Autodesk Inventor part; units mm, degrees
ref_plane "YZ Plane" through (0, 0, 0) normal (1, 0, 0) x (0, 1, 0)
ref_plane "XZ Plane" through (0, 0, 0) normal (0, 1, 0) x (-1, 0, 0)
ref_plane "XY Plane" through (0, 0, 0) normal (0, 0, 1) x (1, 0, 0)
sketch "Sketch1" plane through (0, 0, 0) normal (0, 1, 0) x (-1, 0, 0)
  line L0 (0, 0) -> (0, -100)
  line L1 (0, -100) -> (20, -100)
  line L2 (20, -100) -> (20, 0)
  line L3 (20, 0) -> (0, 0)
  point P0 (10, -5)
  point P1 (10, -95)
  dimension "d0" = 100
  dimension "d1" = 20
  dimension "d2" = 90
  dimension "d3" = 5
extrude "Extrusion1" add sketch "Sketch1" along normal blind 5.5
hole "Hole1" at (-10, 0, -5) at (-10, 0, -95) direction (0, 1, 0) diameter 5.9175 depth 19.1 tip angle 118
properties part number "CB"
Design review of the part built by this model. Coordinates are the model's own, in mm. Give positions to 0.01 mm unless a question says otherwise; leave off trailing zeros. Order: outer loops, then holes, each group sorted by start corner. A loop starts at its lowest first (then second) coordinate and runs counter-clockwise, first axis right, second up. Notation, with made-up numbers: (25.5, -28.75) - (36.5, -28.75) arc R10 ccw to (36.5, -16.75) - close; hole circle Ø2 at (47, -9). An arc over 180 degrees is marked (long way). Use CSV: the item, a comma, the result in double quotes. Start each with the question number.
Q1. Take a section at C-C (y = 4.25). State the section outline as (x, z) points, and give its area (4 significant figures).
Q2. For P1, Ø5.5, axis at x = -10, z = -5, coming from the +Y side, flat-tipped, find the tip position at first contact; note if it passes through.
Q3. Take a section at B-B (z = -5). State the section outline as (x, y) points.
Q4. For line 1 (Z direction, x = -10, y = 2.05); line 2 (X direction, y = 3.2, z = -95); line 3 (Z direction, x = -12.25, y = 5.25), list the stretches that pass through material, from the lowest coordinate up.
Q5. Take a section at A-A (x = -10). State the section outline as (y, z) points.
Q6. Draft analysis for pull direction Z (two halves, no side actions). For faces 1 (the face through (0, 3, -49)), 2 (the face through (-10, 3, -100)), 3 (the face through (-12, 2.79, -2.82)), state which applies: pulls with the +Z half, pulls with the -Z half, needs draft (parallel to the pull), parting line crosses it, or undercut.
Calculated:
1,outline,"(-20, -100) - (0, -100) - (0, 0) - (-20, 0) - close; hole circle Ø5.92 at (-10, -95); hole circle Ø5.92 at (-10, -5)"
1,area,"1,945 mm²"
2,P1,"passes through"
3,outline,"(-20, 0) - (-12.96, 0) - (-12.96, 5.5) - (-20, 5.5) - close; (-7.04, 0) - (0, 0) - (0, 5.5) - (-7.04, 5.5) - close"
4,line 1,"z = -100 to -97.96, -92.04 to -7.96, -2.04 to 0"
4,line 2,"x = -20 to -12.96, -7.04 to 0"
4,line 3,"z = -100 to -96.92, -93.08 to -6.92, -3.08 to 0"
5,outline,"(0, -100) - (5.5, -100) - (5.5, -97.96) - (0, -97.96) - close; (0, -92.04) - (5.5, -92.04) - (5.5, -7.96) - (0, -7.96) - close; (0, -2.04) - (5.5, -2.04) - (5.5, 0) - (0, 0) - close"
6,face 1,"needs draft"
6,face 2,"pulls with the -Z half"
6,face 3,"undercut"
